The figure shows three views and two pictorial views of one solid part (mm, origin at its lowest corner). Answer the questions. Round coordinates to 2 decimals unless told otherwise and drop trailing zeros. Loops run counter-clockwise (first coordinate to the right, second up) from the corner with the lowest first, then second, coordinate; pieces in that order, holes last. Notation, with made-up numbers: (24.25, 56) -> (60.25, 56) arc R16 cw to (60.25, 85) -> close; hole circle Ø2 at (65, -7.5). An arc over 180 degrees is marked (long way). Use a Markdown table: item, result. Add a question column.
Q1. Given pin 1 Ø3.5 at (x, z) = (20, 22.5) entering from -Y; pin 2 Ø1.5 at (y, z) = (3, 17) entering from +X; pin 3 Ø5 at (x, z) = (50, 6.5) entering from -Y, each flat-ended and moving along its own axis, determine where each tip first touches the part or whether it passes through.
Q2. For a pull along Z with two mould halves and no side action, classify the marked faces 1, 2 and 3 as released by +Z, released by -Z, zero draft, split by the parting line, or undercut.
Q3. Section D-D on x = 34 is taken. Give the vertices of the cut face in (y, z) (3 decimals), then the cut area to 3 significant figures.
Q4. Section C-C on z = 6.5 is taken. Give the vertices of the cut face in (x, y), then the cut area to 3 significant figures.
Q5. Section A-A on x = 50 is taken. Give the vertices of the cut face in (y, z), then the cut area to 3 significant figures.
Q6. Consider line 1 (X direction, y = 2.1, z = 22.5); line 2 (X direction, y = 10.25, z = 28.5); line 3 (X direction, y = 10, z = 15.5). Determine where each line is inside the solid, lowest interval first.
Q7. Section B-B on y = 10.5 is taken. Give the number of separate pieces and of enclosed holes in the cut face, then the cut area to 3 significant figures.
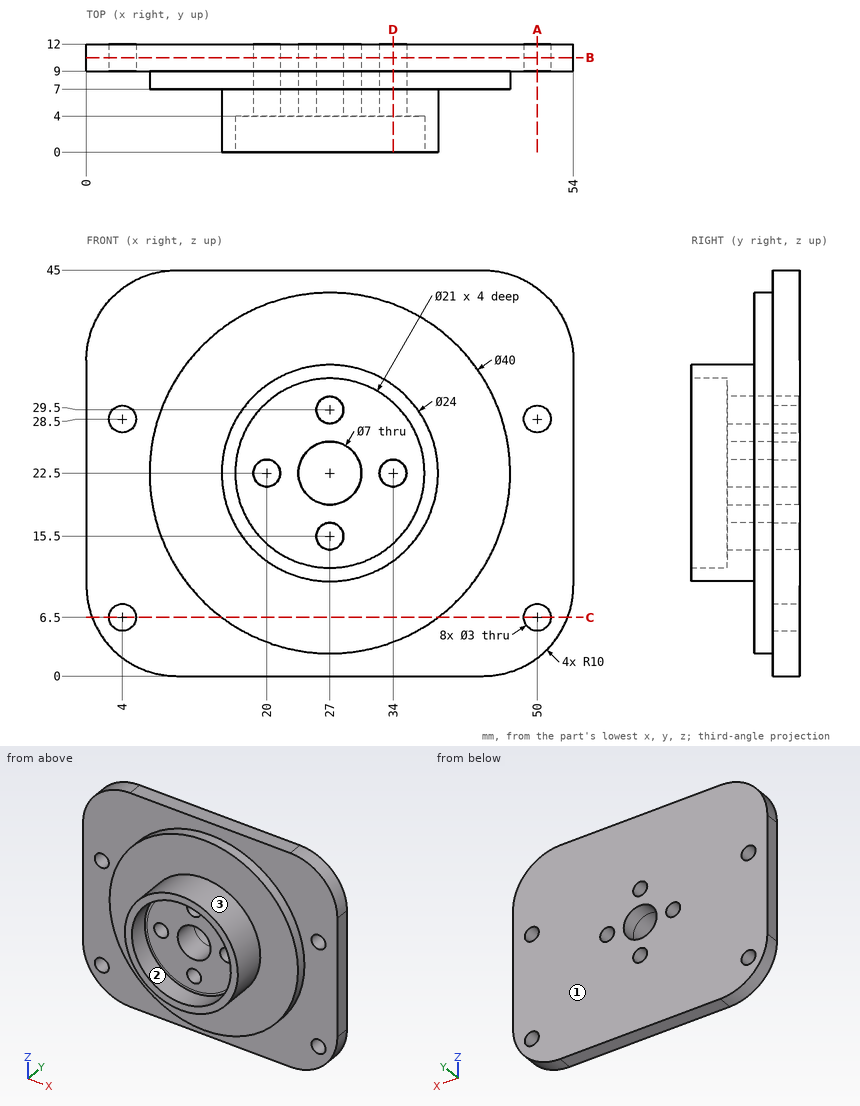
Checked values:
| question | item | result |
|---|---|---|
| 1 | pin 1 | stops at y = 4 |
| 1 | pin 2 | stops at x = 38.02 |
| 1 | pin 3 | stops at y = 9 |
| 2 | face 1 | zero draft |
| 2 | face 2 | undercut |
| 2 | face 3 | split by the parting line |
| 3 | outline | (0, 12.753) -> (7, 12.753) -> (7, 3.765) -> (9, 3.765) -> (9, 0) -> (12, 0) -> (12, 21) -> (4, 21) -> (4, 14.674) -> (0, 14.674) -> close; (0, 30.326) -> (4, 30.326) -> (4, 24) -> (12, 24) -> (12, 45) -> (9, 45) -> (9, 41.235) -> (7, 41.235) -> (7, 32.247) -> (0, 32.247) -> close |
| 3 | area | 260 mm2 |
| 4 | outline | (0.63, 9) -> (2.5, 9) -> (2.5, 12) -> (0.63, 12) -> close; (5.5, 9) -> (15, 9) -> (15, 7) -> (39, 7) -> (39, 9) -> (48.5, 9) -> (48.5, 12) -> (5.5, 12) -> close; (51.5, 9) -> (53.37, 9) -> (53.37, 12) -> (51.5, 12) -> close |
| 4 | area | 188 mm2 |
| 5 | outline | (9, 2) -> (12, 2) -> (12, 5) -> (9, 5) -> close; (9, 8) -> (12, 8) -> (12, 27) -> (9, 27) -> close; (9, 30) -> (12, 30) -> (12, 43) -> (9, 43) -> close |
| 5 | area | 105 mm2 |
| 6 | line 1 | x = 15 to 16.5, 37.5 to 39 |
| 6 | line 2 | x = 0 to 2.5, 5.5 to 25.88, 28.12 to 48.5, 51.5 to 54 |
| 6 | line 3 | x = 0 to 25.5, 28.5 to 54 |
| 7 | separate pieces | 1 |
| 7 | enclosed holes | 9 |
| 7 | area | 2,250 mm2 |
